Check sheet for the modelled part. Datum: model origin and axes. Units: mm. A direction names the side the tool comes from. Coordinates: 2 decimals unless noted, no trailing zeros. Loops run counter-clockwise (first coordinate to the right, second up) from the corner with the lowest first, then second, coordinate; pieces in that order, holes last. Notation, with made-up numbers: (45.5, 82.5) -> (100.5, 82.5) arc R19 cw to (100.5, 87.5) -> close; hole circle Ø11 at (75, 54.5). An arc over 180 degrees is marked (long way). Use one line per item in the form item = value.
from build123d import *

# Parameters (mm, degrees)
SKETCH1_W           = 12.7
SKETCH1_H           = 76.2
SKETCH1_W_2         = 190.5
BOSS_EXTRUDE1_DEPTH = 25.4


with BuildPart() as part:
    # Sketch1 → Boss-Extrude1 (new body)
    with BuildSketch(Plane(origin=(0, 0, 0), x_dir=(0, 0, -1), z_dir=(1, 0, 0))):
        Polygon((95.25, 191.38745187), (-95.25, 181.62487678), (-95.25, 38.1), (95.25, 38.1), align=None)
        with Locations((101.6, 0)):
            Rectangle(SKETCH1_W, SKETCH1_H)
        Rectangle(SKETCH1_W_2, SKETCH1_H)
        with Locations((-101.6, 0)):
            Rectangle(SKETCH1_W, SKETCH1_H)
        Polygon((95.25, -38.1), (-95.25, -38.1), (-95.25, -132.320724436), (95.25, -164.508767502), align=None)
    extrude(amount=BOSS_EXTRUDE1_DEPTH)


solid = part.part
(1) Section check A-A, the plane x = 6. Record the boundary of the cut face in (y, z), plus the area to 3 significant figures.
Established:
outline = (-164.51, -95.25) -> (-38.1, -95.25) -> (-38.1, -107.95) -> (38.1, -107.95) -> (38.1, -95.25) -> (191.39, -95.25) -> (181.62, 95.25) -> (38.1, 95.25) -> (38.1, 107.95) -> (-38.1, 107.95) -> (-38.1, 95.25) -> (-132.32, 95.25) -> close
area = 65,700 mm²
(2) Go/stop test with flat-tipped pins: P1, Ø12.5, axis at x = 18.5, y = 80.5, coming from the -Z side; P2, Ø12.5, axis at x = 9.5, y = 122, coming from the +Z side; P3, Ø6.5, axis at x = 12.5, z = 102.5, coming from the -Y side. Record where each tip stops, or that it passes through.
Established:
P1 = -95.25
P2 = 95.25
P3 = -38.1
(3) Tool access check on faces 1 (the flat face through (13, 38.1, -102)), 2 (the flat face through (13, -102, -95.25)), 3 (the flat face through (13, 111, 95.25)), 4 (the flat face through (13, -1, 107.95)), 5 (the flat face through (13, -85, 95.25)). Record the directions out of +Z, -Z, +X, -X, +Y, -Y that give a thin tool (end or side, any length) a straight path to the whole face; none if there is none.
Established:
face_1 = -Z, +X, -X, +Y
face_2 = -Z, +X, -X, -Y
face_3 = +Z, +X, -X, +Y
face_4 = +Z, +X, -X, +Y, -Y
face_5 = +Z, +X, -X, -Y
(4) Mould release check, pull along Z, two halves, no side actions. Record for faces 6 (the flat face through (0, 16, 2)), 7 (the flat face through (12.52, -148.19, 1.33)), 8 (the flat face through (13, -1, -107.95)): +Z half, -Z half, draft (parallel to the pull), parting line (faces both ways), or undercut.
Established:
face_6 = draft
face_7 = +Z half
face_8 = -Z half
(5) Section check B-B, the plane y = -86. Record the boundary of the cut face in (x, z).
Established:
outline = (0, -95.25) -> (25.4, -95.25) -> (25.4, 95.25) -> (0, 95.25) -> close
(6) Scan lines: line 1 along Z through (x, y) = (10.5, 85); line 2 along Y through (x, z) = (16, -5.5); line 3 along Y through (x, z) = (15.75, -54.5). Record each from-to range of solid material in increasing order.
Established:
line_1 = -95.25 to 95.25
line_2 = -149.34 to 186.79
line_3 = -157.62 to 189.3
(7) Section check C-C, the plane z = -51. Record the boundary of the cut face in (x, y).
Established:
outline = (0, -157.03) -> (25.4, -157.03) -> (25.4, 189.12) -> (0, 189.12) -> close
